```python
from build123d import *

# Parameters (mm, degrees)
BOSS_EXTRUDE1_DEPTH = 40
SKETCH2_R           = 5
BOSS_EXTRUDE2_DEPTH = 500


with BuildPart() as part:
    # Sketch1 → Boss-Extrude1 (new body)
    with BuildSketch(Plane.XY):
        Polygon((184.521008641, -60.40023797), (39.952363844, 190), (-39.952363844, 190), (-184.521008641, -60.40023797), (-144.568644797, -129.59976203), (144.568644797, -129.59976203), align=None)
    boss_extrude1 = extrude(amount=-BOSS_EXTRUDE1_DEPTH)

    # Sketch2 → Boss-Extrude2 (add)
    with BuildSketch(Plane.XY):
        with Locations((25, 157.841136245)):
            Circle(SKETCH2_R)
        with Locations((-25, 157.841136245)):
            Circle(SKETCH2_R)
        with Locations((124.19443375, -100.571203217)):
            Circle(SKETCH2_R)
        with Locations((149.19443375, -57.269933028)):
            Circle(SKETCH2_R)
        with Locations((-149.19443375, -57.269933028)):
            Circle(SKETCH2_R)
        with Locations((-124.19443375, -100.571203217)):
            Circle(SKETCH2_R)
    extrude(amount=BOSS_EXTRUDE2_DEPTH)

    # Mirror1: Boss-Extrude1 across plane
    add(boss_extrude1.mirror(Plane.XY.offset(250)))


solid = part.part
```
Model file for the job. Use its own axes, mm. Coordinates: 2 decimals unless noted, no trailing zeros. Order: outer loops, then holes, each group sorted by start corner. A loop starts at its lowest first (then second) coordinate and runs counter-clockwise, first axis right, second up. Notation, with made-up numbers: (53, 82.5) -> (73, 82.5) arc R13 cw to (73, 105.5) -> close; hole circle Ø11 at (-4, 1). An arc over 180 degrees is marked (long way). Answer as a JSON object with one key per item and string values. Group by question number.
1) Drill centre lines: L1, parallel to Z at x = -1.5, y = 79.5; L2, parallel to Y at x = 24, z = 406; L3, parallel to X at y = 56, z = -15.5. Where is each one in solid material? Low to high.
2) Cut at C-C, the plane z = 59. Write the cut outline in (x, y), then the cut area to 3 significant figures.
3) Cut at A-A, the plane y = -72. Write the cut outline in (x, z).
4) Pull direction Z, two halves, no side cores. Call faces 1 (the face through (-3, -3, 500)), 2 (the face through (-3, -3, 540)), 3 (the face through (113.249, 63.047, 519.72)): +Z half, -Z half, draft (parallel to the pull), parting line (faces both ways), or undercut.
5) Flat gauge pins, fed straight in: pin 1 (8 mm diameter, centred on x = 120, z = 262, fed in from +Y) (3 decimals); pin 2 (2 mm diameter, centred on x = -19.5, z = 80.5, fed in from +Y); pin 3 (1.5 mm diameter, centred on x = -144, z = 318, fed in from -Y). Where does each tip first touch, or does it go through?
6) Cut at B-B, the plane x = -61. Write the cut outline in (y, z), then the cut area to 3 significant figures.
Check values:
{
 "1": {"L1": "z = -40 to 0, 500 to 540", "L2": "y = 152.94 to 162.74", "L3": "x = -117.32 to 117.32"},
 "2": {"outline": "circle Ø10 at (-149.19, -57.27); circle Ø10 at (-124.19, -100.57); circle Ø10 at (-25, 157.84); circle Ø10 at (25, 157.84); circle Ø10 at (124.19, -100.57); circle Ø10 at (149.19, -57.27)", "area": "471 mm²"},
 "3": {"outline": "(-177.82, -40) -> (177.82, -40) -> (177.82, 0) -> (-177.82, 0) -> close; (-177.82, 500) -> (177.82, 500) -> (177.82, 540) -> (-177.82, 540) -> close"},
 "4": {"face 1": "undercut", "face 2": "+Z half", "face 3": "draft"},
 "5": {"pin 1": "stops at y = -95.575", "pin 2": "stops at y = 160.02", "pin 3": "stops at y = -59.56"},
 "6": {"outline": "(-129.6, -40) -> (153.54, -40) -> (153.54, 0) -> (-129.6, 0) -> close; (-129.6, 500) -> (153.54, 500) -> (153.54, 540) -> (-129.6, 540) -> close", "area": "22,700 mm²"}
}
